Build history of the part. All positions in model axes, mm. Face numbers are marked on the shaded views. A direction names the side the tool comes from. Coordinates: 2 decimals unless noted, no trailing zeros. Order: outer loops, then holes, each group sorted by start corner. A loop starts at its lowest first (then second) coordinate and runs counter-clockwise, first axis right, second up. Notation, with made-up numbers: M -18,37.5 L 27,37.5 A27 ccw 27,66.5 Z; hole C 32,8 d8. An arc over 180 degrees is marked long. Write item = value, one per line. Start each with the question number.
Q1. Band-saw the part on A-A on x = 0. Write the cut outline in (y, z), plus the area to 3 significant figures.
Q2. Band-saw the part on C-C on z = -4. Write the cut outline in (x, y), plus the area to 3 significant figures.
Q3. Pull direction Y, two halves, no side cores. Call the marked faces 1, 2 and 3: released by +Y, released by -Y, zero draft, split by the parting line, or undercut.
Q4. Band-saw the part on D-D on x = 10.5. Write the cut outline in (y, z).
Q5. Drill centre lines: probe 1 along Y at (x, z) = (0, -3.35); probe 2 along X at (y, z) = (0.25, 12); probe 3 along Z at (x, y) = (-6.25, -3.25). Where is each one in solid material? Low to high.
Q6. Band-saw the part on B-B on y = 0. Write the cut outline in (x, z), plus the area to 4 significant figures.
Q7. 3-axis set-ups, long thin cutter, end or side, ignore diameter. For the marked faces 4 and 5: which of +Z, -Z, +X, -X, +Y, -Y reach the whole face in a straight line?
Q8. Pin check, flat tips, straight feed: P1, Ø6, axis at x = 2.5, z = 1, coming from the +Y side; P2, Ø5, axis at x = 10, y = 0, coming from the +Z side; P3, Ø1, axis at y = -1.5, z = 9, coming from the +X side; P4, Ø1.5, axis at y = 6, z = 10, coming from the -X side. Stop position of each tip, or through.
```python
from build123d import *

# Parameters (mm, degrees)
SKETCH1_R           = 7
BOSS_EXTRUDE1_DEPTH = 11.5
SKETCH2_R           = 6
BOSS_EXTRUDE2_DEPTH = 5.5
SKETCH3_R           = 13
SKETCH3_R_2         = 1.5
BOSS_EXTRUDE3_DEPTH = 5.5
SKETCH4_R           = 1.85
CUT_EXTRUDE1_DEPTH  = 30.055980452


with BuildPart() as part:
    # Sketch1 → Boss-Extrude1 (new body)
    with BuildSketch(Plane.XY):
        Circle(SKETCH1_R)
    extrude(amount=BOSS_EXTRUDE1_DEPTH)

    # Sketch2 → Boss-Extrude2 (add)
    with BuildSketch(Plane.XY.offset(11.5)):
        Circle(SKETCH2_R)
    extrude(amount=BOSS_EXTRUDE2_DEPTH)

    # Sketch3 → Boss-Extrude3 (add)
    with BuildSketch(Plane(origin=(0, 0, 0), x_dir=(-1, 0, 0), z_dir=(0, 0, -1))):
        Circle(SKETCH3_R)
        with Locations((10, 0)):
            Circle(SKETCH3_R_2, mode=Mode.SUBTRACT)
        with Locations((0, -10)):
            Circle(SKETCH3_R_2, mode=Mode.SUBTRACT)
        with Locations((-10, 0)):
            Circle(SKETCH3_R_2, mode=Mode.SUBTRACT)
        with Locations((0, 10)):
            Circle(SKETCH3_R_2, mode=Mode.SUBTRACT)
    extrude(amount=BOSS_EXTRUDE3_DEPTH)

    # Sketch4 → Cut-Extrude1 (cut, through all)
    with BuildSketch(Plane.XY.offset(17)):
        with Locations((3.6, -3.04e-07)):
            Circle(SKETCH4_R)
        with Locations((-3.6, 0)):
            Circle(SKETCH4_R)
    extrude(amount=-CUT_EXTRUDE1_DEPTH, mode=Mode.SUBTRACT)


solid = part.part
```
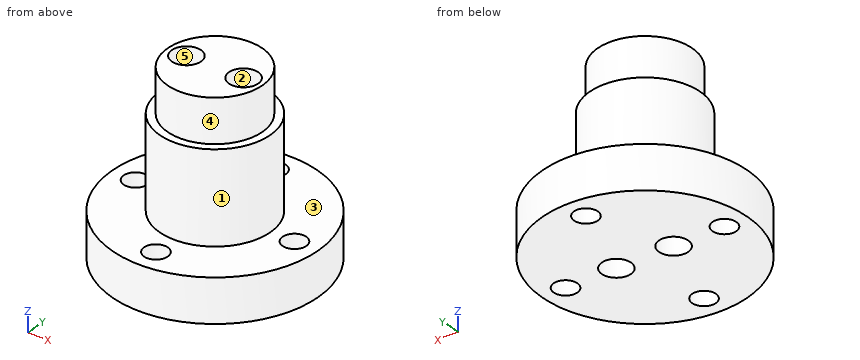
Recorded:
q1.outline = M -13,-5.5 L -11.5,-5.5 L -11.5,0 L -13,0 Z; M -8.5,-5.5 L 8.5,-5.5 L 8.5,0 L 7,0 L 7,11.5 L 6,11.5 L 6,17 L -6,17 L -6,11.5 L -7,11.5 L -7,0 L -8.5,0 Z; M 11.5,-5.5 L 13,-5.5 L 13,0 L 11.5,0 Z
q1.area = 337 mm2
q2.outline = C 0,0 d26; hole C -10,0 d3; hole C -3.6,0 d3.7; hole C 0,-10 d3; hole C 0,10 d3; hole C 3.6,0 d3.7; hole C 10,0 d3
q2.area = 481 mm2
q3.face_1 = split by the parting line
q3.face_2 = undercut
q3.face_3 = zero draft
q4.outline = M -7.66,-5.5 L -1.41,-5.5 L -1.41,0 L -7.66,0 Z; M 1.41,-5.5 L 7.66,-5.5 L 7.66,0 L 1.41,0 Z
q5.probe_1 = -13 to -11.5, -8.5 to 8.5, 11.5 to 13
q5.probe_2 = -5.99 to -5.43, -1.77 to 1.77, 5.43 to 5.99
q5.probe_3 = -5.5 to 0
q6.outline = M -13,-5.5 L -11.5,-5.5 L -11.5,0 L -13,0 Z; M -8.5,-5.5 L -5.45,-5.5 L -5.45,17 L -6,17 L -6,11.5 L -7,11.5 L -7,0 L -8.5,0 Z; M -1.75,-5.5 L 1.75,-5.5 L 1.75,17 L -1.75,17 Z; M 5.45,-5.5 L 8.5,-5.5 L 8.5,0 L 7,0 L 7,11.5 L 6,11.5 L 6,17 L 5.45,17 Z; M 11.5,-5.5 L 13,-5.5 L 13,0 L 11.5,0 Z
q6.area = 170.5 mm2
q7.face_4 = +Z
q7.face_5 = +Z, -Z
q8.P1 = 13
q8.P2 = 0
q8.P3 = 6.93
q8.P4 = -4.63
